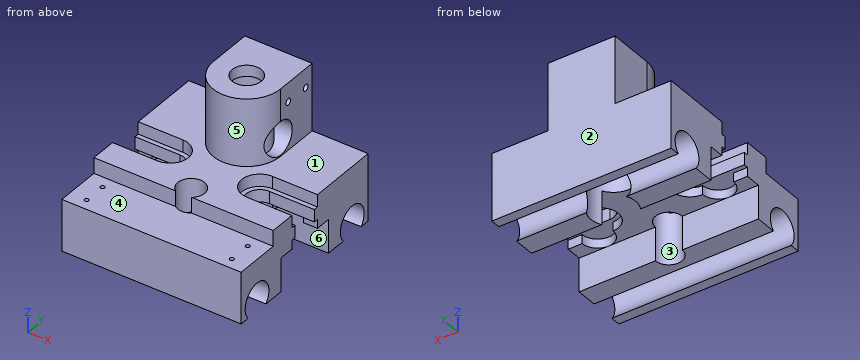
Autodesk Inventor part; units mm, degrees
ref_plane "YZ Plane" through (0, 0, 0) normal (1, 0, 0) x (0, 1, 0)
ref_plane "XZ Plane" through (0, 0, 0) normal (0, 1, 0) x (-1, 0, 0)
ref_plane "XY Plane" through (0, 0, 0) normal (0, 0, 1) x (1, 0, 0)
sketch "Sketch1" plane through (0, 0, 0) normal (0, 0, 1) x (1, 0, 0)
  line L0 (0, 0) -> (80, 0)
  line L1 (80, 0) -> (80, -80)
  line L2 (80, -80) -> (0, -80)
  line L3 (0, -80) -> (0, 0)
  dimension "d0" = 80
  dimension "d1" = 80
extrude "Extrusion1" add sketch "Sketch1" along normal blind 15
sketch "Sketch2" plane through (0, 0, 0) normal (0, 0, -1) x (-1, 0, 0)
  line L0 (0, 0) -> (-80, 0)
  circle A0 centre (-60, -40) radius 6.1
  line L1 (-80, 0) -> (-80, -80)
  line L2 (-60, -33.9) -> (-80, -33.9)
  line L3 (-80, -80) -> (-80, 0)
  line L4 (-60, -46.1) -> (-80, -46.1)
  line L5 (-80, -46.1) -> (-80, -33.9)
  dimension "d7" = 40
  dimension "d8" = 20
  dimension "d9" = 12.2
extrude "Extrusion2" cut sketch "Sketch2" against normal through all
sketch "Sketch3" plane through (0, 0, 0) normal (0, 0, -1) x (-1, 0, 0)
  arc A0 (-60, -46.1) -> (-60, -33.9) centre (-60, -40) ccw
  circle A1 centre (-60, -40) radius 8.1
  line L0 (-60, -31.9) -> (-80, -31.9)
  line L1 (-80, -33.9) -> (-80, 0)
  line L2 (-60, -48.1) -> (-80, -48.1)
  line L3 (-80, -48.1) -> (-80, -31.9)
  point P0 (0, 0)
  dimension "d12" = 16.2
extrude "Extrusion3" cut sketch "Sketch3" against normal blind 4
sketch "Sketch4" plane through (0, 0, 15) normal (0, 0, 1) x (1, 0, 0)
  line L0 (80, -31.9) -> (60, -31.9)
  arc A0 (60, -31.9) -> (60, -48.1) centre (60, -40) ccw
  line L1 (60, -48.1) -> (80, -48.1)
  line L2 (80, -46.1) -> (60, -46.1)
  arc A1 (60, -33.9) -> (60, -46.1) centre (60, -40) ccw
  line L3 (60, -33.9) -> (80, -33.9)
  line L4 (80, -33.9) -> (80, -31.9)
  line L5 (80, -33.9) -> (80, 0)
  line L6 (80, -46.1) -> (80, -48.1)
  line L7 (80, -80) -> (80, -46.1)
  point P0 (0, 0)
extrude "Extrusion4" cut sketch "Sketch4" against normal blind 5.5
sketch "Sketch5" plane through (0, 0, 0) normal (0, 0, -1) x (-1, 0, 0)
  arc A0 (-60, -46.1) -> (-60, -33.9) centre (-60, -40) ccw
  line L0 (-80, -31.9) -> (-60, -31.9)
  circle A1 centre (-60, -40) radius 8.1
  line L1 (-60, -31.9) -> (-60, -31.9)
  line L2 (-73.8, -31.9) -> (-73.8, -48.1)
  line L3 (-60, -48.1) -> (-60, -48.1)
  arc A2 (-60, -48.1) -> (-60, -31.9) centre (-60, -40) ccw
  line L4 (-60, -31.9) -> (-60, -31.9)
  line L5 (-60, -31.9) -> (-60, -31.9)
  line L6 (-60, -33.9) -> (-60, -46.1)
  arc A3 (-60, -31.9) -> (-73.8, -31.9) centre (-66.9, -31.9) ccw
  arc A4 (-73.8, -48.1) -> (-60, -48.1) centre (-66.9, -48.1) ccw
  point P0 (0, 0)
  dimension "d17" = 13.8
  dimension "d20" = 16.2
  dimension "d21" = 8.1
  dimension "d37" = 0
extrude "Extrusion5" cut sketch "Sketch5" against normal blind 4 contours A3 L0 | L0 A1 A4 L2
sketch "Sketch6" plane through (80, 0, 15) normal (1, 0, 0) x (0, 0, -1)
  line L0 (15, 0) -> (0, 0)
  line L1 (15, 0) -> (30, 0)
  line L2 (30, -25) -> (15, -25)
  line L3 (15, -25) -> (15, 0)
  line L4 (15, -80) -> (0, -80)
  line L5 (15, -80) -> (30, -80)
  line L6 (30, -55) -> (15, -55)
  line L7 (15, -55) -> (15, -80)
  arc A0 (30, -4.4098) -> (30, -15.5902) centre (25, -10) ccw
  arc A1 (30, -64.4098) -> (30, -75.5902) centre (25, -70) ccw
  line L8 (30, 0) -> (30, -4.4098)
  line L9 (30, -15.5902) -> (30, -25)
  line L10 (30, -80) -> (30, -75.5902)
  line L11 (30, -64.4098) -> (30, -55)
  dimension "d22" = 25
  dimension "d23" = 25
  dimension "d24" = 15
  dimension "d25" = 15
  dimension "d29" = 15
  dimension "d32" = 15
  dimension "d33" = 5
  dimension "d34" = 5
  dimension "d38" = 15
  dimension "d39" = 15
  dimension "d40" = 60
  dimension "d41" = 10
  dimension "d42" = 10
extrude "Extrusion6" add sketch "Sketch6" against normal blind 80
ref_plane "Work Plane1" through (40, -33.9, 4) normal (1, 0, 0) x (0, 0, -1)
mirror "Mirror1" about plane through (40, -33.9, 4) normal (1, 0, 0) of "Extrusion5", "Extrusion4", "Extrusion3", "Extrusion2"
sketch "Sketch8" plane through (80, -48.1, 4) normal (1, 0, 0) x (0, 0, -1)
  line L0 (-11, 0) -> (-11, -31.9)
  line L1 (-11, -31.9) -> (-4, -31.9)
  line L2 (-4, -31.9) -> (-4, -11.7)
  line L3 (-4, -11.7) -> (-11, -11.7)
  line L4 (-11, -11.7) -> (-11, -31.9)
  point P0 (4, 48.1)
  dimension "d49" = 20.2
  dimension "d50" = 7
extrude "Extrusion8" cut sketch "Sketch8" along normal through all both and the other way through all
sketch "Sketch9" plane through (80, -80, 8) normal (0, 0, 1) x (1, 0, 0)
  circle A0 centre (-7.6, 14.9) radius 0.95
  circle A1 centre (-7.6, 4.9) radius 0.95
  line L0 (0, 20.2) -> (0, 0)
  line L1 (0, 0) -> (-80, 0)
  point P0 (-80, 80)
  dimension "d53" = 1.9
  dimension "d54" = 1.9
  dimension "d55" = 7.6
  dimension "d56" = 7.6
  dimension "d57" = 10
  dimension "d58" = 4.9
extrude "Extrusion9" cut sketch "Sketch9" against normal blind 10
ref_plane "Work Plane2" through (40, -48.1, 4) normal (1, 0, 0) x (0, 0, -1)
mirror "Mirror2" about plane through (40, -48.1, 4) normal (1, 0, 0) of "Extrusion9"
sketch "Sketch10" plane through (0, 0, 15) normal (0, 0, 1) x (1, 0, 0)
  line L0 (80, -55) -> (0, -55)
  circle A0 centre (40, -55) radius 6
  point P0 (0, 0)
  dimension "d61" = 12
extrude "Extrusion10" cut sketch "Sketch10" against normal through all
sketch "Sketch11" plane through (0, 0, 15) normal (0, 0, 1) x (1, 0, 0)
  circle A0 centre (40, -20) radius 15
  circle A1 centre (40, -20) radius 10
  line L0 (80, -31.9) -> (80, 0)
  line L1 (80, 0) -> (0, 0)
  line L2 (55, -20) -> (55, -5)
  line L3 (80, -4.4098) -> (0, -4.4098)
  line L4 (55, -5) -> (40, -5)
  line L5 (40, -5) -> (25, -5)
  line L6 (25, -5) -> (25, -20)
  line L7 (55, -5) -> (25, -5)
  line L8 (25, -5) -> (25, 0)
  line L9 (25, 0) -> (55, 0)
  line L10 (55, 0) -> (55, -5)
  dimension "d64" = 30
  dimension "d65" = 20
  dimension "d66" = 40
  dimension "d67" = 20
extrude "Extrusion11" add sketch "Sketch11" along normal blind 30 contours A0 | A0 L4 L2 | L5 L8 L3 L10 L4 | A0 L6 L5 | L3 L8 L1 L10
sketch "Sketch12" plane through (0, 0, 45) normal (0, 0, 1) x (1, 0, 0)
  circle A0 centre (40, -20) radius 10
  circle A1 centre (40, -20) radius 6.5
  point P0 (0, 0)
  dimension "d70" = 13
extrude "Extrusion12" add sketch "Sketch12" against normal blind 5
sketch "Sketch13" plane through (0, 0, 15) normal (0, 0, 1) x (1, 0, 0)
  circle A0 centre (40, -20) radius 6.5
  circle A1 centre (40, -20) radius 10
  point P0 (0, 0)
extrude "Extrusion13" cut sketch "Sketch13" against normal blind 35 contours A0 | A1
sketch "Sketch14" plane through (55, -20, 15) normal (1, 0, 0) x (0, 0, -1)
  circle A0 centre (-21.5, 5) radius 1.45
  circle A1 centre (-21.5, 16) radius 1.45
  line L0 (0, 20) -> (-30, 20)
  line L1 (-30, 0) -> (-30, 20)
  point P0 (15, 20)
  dimension "d75" = 2.9
  dimension "d76" = 2.9
  dimension "d77" = 11
  dimension "d78" = 4
  dimension "d79" = 8.5
  dimension "d80" = 8.5
extrude "Extrusion14" cut sketch "Sketch14" against normal blind 15
sketch "Sketch15" plane through (55, -20, 15) normal (1, 0, 0) x (0, 0, -1)
  circle A0 centre (-8, 0) radius 7.5
  line L0 (15, -10) -> (-25, -10)
  line L1 (4, -6) -> (-11, -6)
  line L2 (4, 6) -> (-11, 6)
  line L3 (0, -11.9) -> (0, 20)
  point P0 (15, 20)
  dimension "d83" = 6
  dimension "d84" = 15
  dimension "d85" = 8
extrude "Extrusion15" cut sketch "Sketch15" against normal blind 17 contours A0
equation "\"d24\" = d25"
equation "\"d32\" = d29"
equation "\"d34\" = d33"
equation "\"d75\" = d76"
equation "\"d80\" = d79"
equation "\"RodDiameter\" = 8"
equation "\"VerticalBearingOD\" = 16"
equation "\"PrintingClearance\" = 0.2"
equation "\"d31\" = d30"
equation "\"TubeID\" = 18"
properties part number "HotendMountCarriage"
Read the model definition and answer for the solid it produces. Units are mm, in the model's axes. Face numbers are marked on the shaded views. A direction names the side the tool comes from. Coordinates: 2 decimals unless noted, no trailing zeros. Loops run counter-clockwise (first coordinate to the right, second up) from the corner with the lowest first, then second, coordinate; pieces in that order, holes last. Notation, with made-up numbers: (3, 21) -> (28, 21) arc R30 ccw to (28, 51) -> close; hole circle Ø5 at (42, 59). An arc over 180 degrees is marked (long way). Return JSON: item names as keys, results as strings.
Item 1: For the marked faces 4, 5 and 6, determine the directions among +Z, -Z, +X, -X, +Y, -Y from which every point of the face is accessible in a straight line to the end or side of a thin tool.
Answers:
{"face 4": "+Z, +X, -X, -Y", "face 5": "+Z, -Y", "face 6": "-Z, +X, -X"}
Item 2: Find section A-A (z = 12.5). Determine the outline of the cut face in (x, y), plus the area to 3 significant figures.
Answers:
{"outline": "(0, -59.8) -> (36.4, -59.8) arc R6 cw (long way) to (43.6, -59.8) -> (80, -59.8) -> (80, -48.1) -> (60, -48.1) arc R8.1 cw to (60, -31.9) -> (80, -31.9) -> (80, 0) -> (0, 0) -> (0, -31.9) -> (20, -31.9) arc R8.1 cw to (20, -48.1) -> (0, -48.1) -> close; hole circle Ø20 at (40, -20)", "area": "3,510 mm2"}
Item 3: Find section C-C (x = 17). Determine the outline of the cut face in (y, z).
Answers:
{"outline": "(-80, -15) -> (-75.59, -15) arc R7.5 cw (long way) to (-64.41, -15) -> (-55, -15) -> (-55, 0) -> (-53.79, 0) -> (-53.79, 4) -> (-46.1, 4) -> (-46.1, 9.5) -> (-48.1, 9.5) -> (-48.1, 15) -> (-59.8, 15) -> (-59.8, 8) -> (-80, 8) -> close; (-33.9, 4) -> (-26.21, 4) -> (-26.21, 0) -> (-25, 0) -> (-25, -15) -> (-15.59, -15) arc R7.5 cw (long way) to (-4.41, -15) -> (0, -15) -> (0, 15) -> (-31.9, 15) -> (-31.9, 9.5) -> (-33.9, 9.5) -> close"}
Item 4: Find section D-D (z = -9.5). Determine the outline of the cut face in (x, y), plus the area to 3 significant figures.
Answers:
{"outline": "(0, -80) -> (80, -80) -> (80, -77.48) -> (0, -77.48) -> close; (0, -62.52) -> (80, -62.52) -> (80, -55) -> (46, -55) arc R6 cw to (34, -55) -> (0, -55) -> close; (0, -25) -> (31.34, -25) arc R10 cw to (30.32, -17.48) -> (0, -17.48) -> close; (0, -2.52) -> (80, -2.52) -> (80, 0) -> (0, 0) -> close; (48.66, -25) -> (80, -25) -> (80, -17.48) -> (49.68, -17.48) arc R10 cw to start", "area": "1,400 mm2"}
Item 5: For a pull along Y with two mould halves and no side action, classify the marked faces 1, 2 and 3 as +Y half, -Y half, draft (parallel to the pull), parting line (faces both ways), or undercut.
Answers:
{"face 1": "draft", "face 2": "+Y half", "face 3": "undercut"}
Item 6: Find section B-B (y = -57.5). Determine the outline of the cut face in (x, z).
Answers:
{"outline": "(0, -15) -> (34.55, -15) -> (34.55, 15) -> (0, 15) -> close; (45.45, -15) -> (80, -15) -> (80, 15) -> (45.45, 15) -> close"}
Item 7: Find the intervals of material crossed by probe 1 along X at (y, z) = (-65.1, 3.25); probe 2 along Y at (x, z) = (24, -10); probe 3 along X at (y, z) = (-20, -2.5), in increasing order.
Answers:
{"probe 1": "x = 0 to 6.65, 8.55 to 71.45, 73.35 to 80", "probe 2": "y = -80 to -77.5, -62.5 to -55, -25 to -17.5, -2.5 to 0", "probe 3": "x = 0 to 30, 50 to 80"}
Item 8: Flat-ended cylindrical pins translate along their axes: P1, Ø8, axis at x = 57, z = 26, coming from the -Y side; P2, Ø0.6, axis at x = 7.5, y = -65, coming from the +Z side; P3, Ø22, axis at y = -12, z = 31.5, coming from the -X side; P4, Ø8, axis at x = 60.5, y = -39.5, coming from the +Z side. Find the tip coordinate at first contact, or state that the pin passes through.
Answers:
{"P1": "stops at y = -27.48", "P2": "stops at z = -2", "P3": "stops at x = 25", "P4": "passes through"}
